Design review of the part built by this model. Coordinates are the model's own, in mm. A direction names the side the tool comes from. Give positions to 0.01 mm unless a question says otherwise; leave off trailing zeros. Write each loop counter-clockwise with the first axis right and the second up, starting at its lowest first coordinate (ties: lowest second). Pieces come first, ordered by that corner, then holes. Notation, with made-up numbers: (59, 66.5) -> (66, 66.5) arc R19 cw to (66, 89.5) -> close; hole circle Ø9 at (25.25, 3). An arc over 180 degrees is marked (long way). Answer as a JSON object with one key per item and string values.
```python
from build123d import *

# Parameters (mm, degrees)
BOSS_EXTRU_2_DEPTH = 70
CONG_4_R           = 2
CONG_3_R           = 2
CONG_5_R           = 2
CONG_6_R           = 2
COQUE1_START       = 3
COQUE1_DEPTH       = 64
CONG_7_R           = 2
CONG_8_R           = 2


# Read off the part's stored shape, not the designer's step: Coque1
with BuildPart() as part:
    # Esquisse2 → Boss.-Extru.2 (new body)
    with BuildSketch(Plane.XY):
        Polygon((-35.5, 0), (-20.5, 0), (-20.5, 20), (20.5, 20), (20.5, 0), (35.5, 0), (35.5, 60), (-35.5, 60), align=None)
    extrude(amount=BOSS_EXTRU_2_DEPTH)

    # Congé4
    cong_4_edges = [part.edges().sort_by_distance(p)[0] for p in [
        (-35.5, 60, 35),
    ]]
    fillet(cong_4_edges, radius=CONG_4_R)

    # Congé3
    cong_3_edges = [part.edges().sort_by_distance(p)[0] for p in [
        (35.5, 60, 35),
    ]]
    fillet(cong_3_edges, radius=CONG_3_R)

    # Congé5
    cong_5_edges = [part.edges().sort_by_distance(p)[0] for p in [
        (20.5, 20, 35),
    ]]
    fillet(cong_5_edges, radius=CONG_5_R)

    # Congé6
    cong_6_edges = [part.edges().sort_by_distance(p)[0] for p in [
        (-20.5, 20, 35),
    ]]
    fillet(cong_6_edges, radius=CONG_6_R)

    # Coque1 outline → Coque1 (cut)
    with BuildSketch(Plane.XY.offset(COQUE1_START)):
        with BuildLine():
            Line((-32.5, 60), (-32.5, 3))
            Line((-32.5, 3), (-23.5, 3))
            Line((-23.5, 3), (-23.5, 18))
            ThreePointArc((-23.5, 18), (-22.035533906, 21.535533906), (-18.5, 23))
            Line((-18.5, 23), (18.5, 23))
            ThreePointArc((18.5, 23), (22.035533906, 21.535533906), (23.5, 18))
            Line((23.5, 18), (23.5, 3))
            Line((23.5, 3), (32.5, 3))
            Line((32.5, 3), (32.5, 60))
            Line((32.5, 60), (-32.5, 60))
        make_face()
    extrude(amount=COQUE1_DEPTH, mode=Mode.SUBTRACT)

    # Congé7
    cong_7_edges = [part.edges().sort_by_distance(p)[0] for p in [
        (35.5, 29, 0),
        (34.914213562, 59.414213562, 0),
        (0, 60, 0),
        (-34.914213562, 59.414213562, 0),
        (-28, 0, 0),
        (-35.5, 0, 35),
        (-35.5, 29, 0),
    ]]
    fillet(cong_7_edges, radius=CONG_7_R)

    # Congé8
    cong_8_edges = [part.edges().sort_by_distance(p)[0] for p in [
        (-20.5, 9, 70),
        (35.5, 0, 36),
        (20.5, 0, 35),
        (-20.5, 0, 36),
        (28, 0, 70),
        (35.5, 29, 70),
        (-35.5, 30, 70),
        (-34.914213562, 59.414213562, 70),
        (0, 60, 70),
        (34.914213562, 59.414213562, 70),
        (20.5, 9, 0),
        (20.5, 9, 70),
        (19.914213562, 19.414213562, 0),
        (19.914213562, 19.414213562, 70),
        (0, 20, 0),
        (0, 20, 70),
        (-19.914213562, 19.414213562, 0),
        (-19.914213562, 19.414213562, 70),
        (-20.5, 10, 0),
        (34.914213562, 0, 0.585786438),
        (-27, 0, 70),
        (-20.5, 0.585786438, 0.585786438),
        (-34.914213562, 0.585786438, 70),
        (27, 0, 0),
    ]]
    fillet(cong_8_edges, radius=CONG_8_R)


solid = part.part
```
(1) We need section C-C, the plane y = 43.5. State the section outline as (x, z) points.
Here are the results:
{"outline": "(-35.5, 2) arc R2 ccw to (-33.5, 0) -> (33.5, 0) arc R2 ccw to (35.5, 2) -> (35.5, 68) arc R2 ccw to (33.5, 70) -> (-33.5, 70) arc R2 ccw to (-35.5, 68) -> close; hole (-32.5, 3) -> (32.5, 3) -> (32.5, 67) -> (-32.5, 67) -> close"}
(2) For line 1 along X through (y, z) = (17, 28.5); line 2 along Z through (x, y) = (-2, 51.5); line 3 along X through (y, z) = (40, 23.5), list the stretches that pass through material, from the lowest coordinate up.
Here are the results:
{"line 1": "x = -35.5 to -32.5, -23.5 to -20.5, 20.5 to 23.5, 32.5 to 35.5", "line 2": "z = 0 to 3, 67 to 70", "line 3": "x = -35.5 to -32.5, 32.5 to 35.5"}
(3) Clearance check with flat-ended pins moving along their axes: pin 1 (10 mm diameter, centred on x = 28, z = 45.5, fed in from +Y); pin 2 (12 mm diameter, centred on x = 26, z = 44, fed in from +Y); pin 3 (3 mm diameter, centred on x = 2.5, z = 31.5, fed in from -Y); pin 4 (2 mm diameter, centred on x = -2, y = 20.5, fed in from +Z). State where each tip first meets the part, or that it passes through.
Here are the results:
{"pin 1": "stops at y = 60", "pin 2": "stops at y = 22.77", "pin 3": "stops at y = 20", "pin 4": "stops at z = 69.94"}
(4) The part is to be moulded in two halves that separate along Z. For faces 4 (the flat face through (0, 37, 70)), 5 (the cylindrical face through (-34.9, 0.57, 35.46)), 6 (the cylindrical face through (-34.9, 29.61, 0.57)), 7 (the flat face through (-28, 3, 35)), say which applies: +Z half, -Z half, draft (parallel to the pull), parting line (faces both ways), or undercut.
Here are the results:
{"face 4": "+Z half", "face 5": "draft", "face 6": "-Z half", "face 7": "undercut"}
(5) We need section D-D, the plane x = -17. State the section outline as (y, z) points.
Here are the results:
{"outline": "(20, 2) arc R2 ccw to (22, 0) -> (58, 0) arc R2 ccw to (60, 2) -> (60, 3) -> (23, 3) -> (23, 67) -> (60, 67) -> (60, 68) arc R2 ccw to (58, 70) -> (22, 70) arc R2 ccw to (20, 68) -> close"}
(6) We need section B-B, the plane z = 45.5. State the section outline as (x, y) points, then the cut area to 3 significant figures.
Here are the results:
{"outline": "(-35.5, 2) arc R2 ccw to (-33.5, 0) -> (-22.5, 0) arc R2 ccw to (-20.5, 2) -> (-20.5, 18) arc R2 cw to (-18.5, 20) -> (18.5, 20) arc R2 cw to (20.5, 18) -> (20.5, 2) arc R2 ccw to (22.5, 0) -> (33.5, 0) arc R2 ccw to (35.5, 2) -> (35.5, 58) arc R2 ccw to (33.5, 60) -> (32.5, 60) -> (32.5, 3) -> (23.5, 3) -> (23.5, 18) arc R5 ccw to (18.5, 23) -> (-18.5, 23) arc R5 ccw to (-23.5, 18) -> (-23.5, 3) -> (-32.5, 3) -> (-32.5, 60) -> (-33.5, 60) arc R2 ccw to (-35.5, 58) -> close", "area": "661 mm²"}
(7) For faces 1 (the cylindrical face through (-21.07, 9.89, 0.6)), 2 (the flat face through (20.5, 10, 35)), 3 (the cylindrical face through (-21.07, 10.11, 69.4)), list the 3-axis set-ups (+Z, -Z, +X, -X, +Y, -Y) from which the entire face can be reached by the end or side of a thin tool; tool diameter is ignored.
Here are the results:
{"face 1": "-Z, -Y", "face 2": "+Z, -Z, -Y", "face 3": "+Z, -Y"}
(8) We need section A-A, the plane y = 4. State the section outline as (x, z) points, then the cut area to 3 significant figures.
Here are the results:
{"outline": "(-35.5, 2) arc R2 ccw to (-33.5, 0) -> (-22.5, 0) arc R2 ccw to (-20.5, 2) -> (-20.5, 68) arc R2 ccw to (-22.5, 70) -> (-33.5, 70) arc R2 ccw to (-35.5, 68) -> close; (20.5, 2) arc R2 ccw to (22.5, 0) -> (33.5, 0) arc R2 ccw to (35.5, 2) -> (35.5, 68) arc R2 ccw to (33.5, 70) -> (22.5, 70) arc R2 ccw to (20.5, 68) -> close; hole (-32.5, 3) -> (-23.5, 3) -> (-23.5, 67) -> (-32.5, 67) -> close; hole (23.5, 3) -> (32.5, 3) -> (32.5, 67) -> (23.5, 67) -> close", "area": "941 mm²"}
